```python
from build123d import *

# Parameters (mm, degrees)
F1_DEPTH = 81
F2_R     = 2.5
F3_DEPTH = 51.336541
F5_DEPTH = 100
F6_R     = 4.165
F7_DEPTH = 40


with BuildPart() as f1:
    # F0 (on Front) → F1 (new body)
    with BuildSketch(Plane.XZ):
        Polygon((-12.655995, 51.335541), (-82.655995, 51.335541), (-82.655995, -48.664459), (-24.655995, -48.664459), (-24.655995, 1.335541), (-12.655995, 1.335541), align=None)
    extrude(amount=F1_DEPTH)

    # F2 (on Top) → F3 (cut, through all)
    with BuildSketch(Plane.XY):
        with Locations((-18.655995, -30)):
            Circle(F2_R)
        with Locations((-18.655995, -51)):
            Circle(F2_R)
    extrude(amount=F3_DEPTH, mode=Mode.SUBTRACT)

    # F4 (on Right) → F5 (cut)
    with BuildSketch(Plane.YZ):
        with BuildLine():
            Line((-36.335, 31.335541), (-36.335, 51.335541))
            ThreePointArc((-36.335, 51.335541), (-40.5, 55.500541), (-44.665, 51.335541))
            Line((-44.665, 51.335541), (-44.665, 31.335541))
            ThreePointArc((-44.665, 31.335541), (-40.5, 27.170541), (-36.335, 31.335541))
        make_face()
    extrude(amount=-F5_DEPTH, mode=Mode.SUBTRACT)

    # F6 (on Front) → F7 (cut)
    with BuildSketch(Plane.XZ):
        with Locations((-19.655995, 31.335541)):
            Circle(F6_R)
    extrude(amount=F7_DEPTH, mode=Mode.SUBTRACT)


solid = f1.part
```
Geometry: final body of the model. Coordinates: model frame, mm. A direction names the side the tool comes from. Round coordinates to 2 decimals unless told otherwise and drop trailing zeros. Order: outer loops, then holes, each group sorted by start corner. A loop starts at its lowest first (then second) coordinate and runs counter-clockwise, first axis right, second up. Notation, with made-up numbers: (63.25, -23) -> (110.25, -23) arc R11 cw to (110.25, -13) -> close; hole circle Ø7 at (42, 51.5). An arc over 180 degrees is marked (long way). Use CSV: the item, a comma, the result in double quotes. Start each with the question number.
1) Section B-B (y = -51). Return the cut outline in (x, z).
2) Material intervals for line 1 along Y through (x, z) = (-19, 45) (3 decimals); line 2 along X through (y, z) = (-51, 41); line 3 along Y through (x, z) = (-42.5, 43.5) (3 decimals), sorted ascending. Write a range as from..to.
3) Draft query along X for faces 1 (the face through (-12.656, -40, 26)), 2 (the face through (-16.27, -29.25, 15.01)), 3 (the face through (-20.64, -52.52, 25.99)), 4 (the face through (-48, -81, 2)). Return one class per face: +X half, -X half, draft (parallel to the pull), parting line (faces both ways), or undercut.
4) Section C-C (x = -69). Return the cut outline in (y, z) (3 decimals).
5) Set-up query: faces 5 (the face through (-48, 0, 2)), 6 (the face through (-47, -36.335, 41)), 7 (the face through (-19, -40, 1.336)), 8 (the face through (-20.56, -15.28, 27.27)), 9 (the face through (-54, -40, -48.664)). Return all of +Z, -Z, +X, -X, +Y, -Y with unobstructed straight access to the full face (end or side cutting, diameter ignored); none if empty.
6) Section D-D (y = -66). Return the cut outline in (x, z).
7) First-contact query: pin 1 Ø15 at (y, z) = (-33.5, -21.5) entering from +X; pin 2 Ø9.5 at (x, y) = (-17.5, -37) entering from -Z. Flat tips, straight axial feed; report the tip coordinate or a pass-through.
8) Section A-A (y = -4.5). Return the cut outline in (x, z) (3 decimals), and give its area (3 significant figures).
Returned:
1,outline,"(-82.66, -48.66) -> (-24.66, -48.66) -> (-24.66, 1.34) -> (-21.16, 1.34) -> (-21.16, 51.34) -> (-82.66, 51.34) -> close; (-16.16, 1.34) -> (-12.66, 1.34) -> (-12.66, 51.34) -> (-16.16, 51.34) -> close"
2,line 1,"y = -81..-53.476, -48.524..-44.665, -36.335..-32.476, -27.524..0"
2,line 2,"x = -82.66..-21.16, -16.16..-12.66"
2,line 3,"y = -81..-44.665, -36.335..0"
3,face 1,"+X half"
3,face 2,"undercut"
3,face 3,"undercut"
3,face 4,"draft"
4,outline,"(-81, -48.664) -> (0, -48.664) -> (0, 51.336) -> (-36.335, 51.336) -> (-36.335, 31.336) arc R4.165 cw to (-44.665, 31.336) -> (-44.665, 51.336) -> (-81, 51.336) -> close"
5,face 5,"+Z, -Z, +X, -X, +Y"
5,face 6,"+Z, +X, -X"
5,face 7,"-Z, +X, +Y, -Y"
5,face 8,"+Y"
5,face 9,"-Z, +X, -X, +Y, -Y"
6,outline,"(-82.66, -48.66) -> (-24.66, -48.66) -> (-24.66, 1.34) -> (-12.66, 1.34) -> (-12.66, 51.34) -> (-82.66, 51.34) -> close"
7,pin 1,"stops at x = -24.66"
7,pin 2,"stops at z = 1.34"
8,outline,"(-82.656, -48.664) -> (-24.656, -48.664) -> (-24.656, 1.336) -> (-12.656, 1.336) -> (-12.656, 51.336) -> (-82.656, 51.336) -> close; hole circle Ø8.33 at (-19.656, 31.336)"
8,area,"6,350 mm²"
